```python
from build123d import *

# Parameters (mm, degrees)
SKETCH1_R           = 12.5
BOSS_EXTRUDE1_DEPTH = 15


with BuildPart() as part:
    # Sketch1 → Boss-Extrude1 (new body, symmetric)
    with BuildSketch(Plane.XY):
        with BuildLine():
            Line((37.628606884, 42), (35.5, 42))
            Line((35.5, 42), (35.5, 40))
            Line((35.5, 40), (-37.5, 40))
            Line((-37.5, 40), (-34.927862315, 0))
            ThreePointArc((-34.927862315, 0), (0, -32.754018227), (34.927862315, 0))
            Line((34.927862315, 0), (36.342538042, 22))
            Line((36.342538042, 22), (45.628606884, 22))
            Line((45.628606884, 22), (45.628606884, 42))
            Line((45.628606884, 42), (37.628606884, 42))
        make_face()
        Circle(SKETCH1_R, mode=Mode.SUBTRACT)
    extrude(amount=BOSS_EXTRUDE1_DEPTH, both=True)

    # Sketch2 → Revolve1 (revolve)
    with BuildSketch(Plane.XY):
        Polygon((-37.5, 722), (-17.5, 722), (-17.5, 712), (-32.5, 712), (-32.5, 172), (0, 172), (0, 40), (-37.5, 40), align=None)
    revolve(axis=Axis((0, 722, 0), (0, -1, 0)))


solid = part.part
```
The model under review builds one solid part; all positions refer to its coordinate system, in mm. A direction names the side the tool comes from. Coordinates: 2 decimals unless noted, no trailing zeros. Order: outer loops, then holes, each group sorted by start corner. A loop starts at its lowest first (then second) coordinate and runs counter-clockwise, first axis right, second up. Notation, with made-up numbers: (78, 68.25) -> (112, 68.25) arc R21 ccw to (112, 80.25) -> close; hole circle Ø11 at (53.5, 43). An arc over 180 degrees is marked (long way). Answer in a Markdown table with one row per item. Add a question column.
Item 1: Clearance check with flat-ended pins moving along their axes: pin 1 (5 mm diameter, centred on x = 39, z = 0, fed in from +Y); pin 2 (4 mm diameter, centred on x = -23, y = 357, fed in from -Z); pin 3 (1.5 mm diameter, centred on y = 478, z = 21, fed in from +X); pin 4 (4 mm diameter, centred on y = 236, z = 5.5, fed in from +X). State where each tip first meets the part, or that it passes through.
Item 2: We need section A-A on x = 0. Write out the cut boundary in (y, z).
Item 3: Machinability: for faces 5 (the cylindrical face through (13.887, 716.93, 10.648)), 6 (the flat face through (14, 712, 14)), 7 (the flat face through (0, 40, -24)), 8 (the flat face through (0, 40, 24)), which of the approach directions +Z, -Z, +X, -X, +Y, -Y give a long, thin tool a straight path to every point of the face, cutting with its end or side? Answer none if there is none.
Item 4: We need section B-B on y = 320.5. Write out the cut boundary in (x, z), plus the area to 3 significant figures.
Item 5: To check wall thickness, follow probe 1 along Z at (x, y) = (0, 495.5); probe 2 along X at (y, z) = (720.25, 0). State the ranges of each line that lie inside material, in increasing order.
Item 6: Mouldability with a two-part tool opening along Y and no side actions: class faces 1 (the flat face through (-8, 722, 16)), 2 (the flat face through (0, 172, 0)), 3 (the flat face through (35.625, 10.846, 0.21)), 4 (the flat face through (3, 13, 15)) as +Y half, -Y half, draft (parallel to the pull), parting line (faces both ways), or undercut.
Final values:
| question | item | result |
|---|---|---|
| 1 | pin 1 | stops at y = 722 |
| 1 | pin 2 | stops at z = -31.07 |
| 1 | pin 3 | stops at x = 31.56 |
| 1 | pin 4 | stops at x = 37.34 |
| 2 | outline | (-32.75, -15) -> (-12.5, -15) -> (-12.5, 15) -> (-32.75, 15) -> close; (12.5, -15) -> (40, -15) -> (40, -37.5) -> (722, -37.5) -> (722, -17.5) -> (712, -17.5) -> (712, -32.5) -> (172, -32.5) -> (172, 32.5) -> (712, 32.5) -> (712, 17.5) -> (722, 17.5) -> (722, 37.5) -> (40, 37.5) -> (40, 15) -> (12.5, 15) -> close |
| 3 | face 5 | +Y |
| 3 | face 6 | none |
| 3 | face 7 | -Z, +X, -X, -Y |
| 3 | face 8 | +Z, +X, -X, -Y |
| 4 | outline | circle Ø75 at (0, 0); hole circle Ø65 at (0, 0) |
| 4 | area | 1,100 mm2 |
| 5 | probe 1 | z = -37.5 to -32.5, 32.5 to 37.5 |
| 5 | probe 2 | x = -37.5 to -17.5, 17.5 to 37.5 |
| 6 | face 1 | +Y half |
| 6 | face 2 | undercut |
| 6 | face 3 | -Y half |
| 6 | face 4 | draft |
